from build123d import *

# Parameters (mm, degrees)
F0_W     = 76.2
F0_H     = 25.4
F1_DEPTH = 25.4
F2_W     = 38.1
F2_H     = 25.4
F3_DEPTH = 12.7
F4_R     = 3.175
F5_DEPTH = 12.7


with BuildPart() as f1:
    # F0 (on Front) → F1 (new body)
    with BuildSketch(Plane.XZ):
        with Locations((38.1, 12.7)):
            Rectangle(F0_W, F0_H)
    extrude(amount=F1_DEPTH)

    # F2 (on face) → F3 (cut)
    with BuildSketch(Plane.XY.offset(25.4)):
        with Locations((50.8, -12.7)):
            Rectangle(F2_W, F2_H)
    extrude(amount=-F3_DEPTH, mode=Mode.SUBTRACT)

    # F4 (on face) → F5 (cut)
    with BuildSketch(Plane.XY.offset(12.7)):
        with Locations((43.815, -13.335)):
            Circle(F4_R)
    extrude(amount=-F5_DEPTH, mode=Mode.SUBTRACT)

    # F6: F1 across plane


with BuildPart() as f1_1:
    add(f1.part)
    add(f1.part.mirror(Plane.XY))


solid = f1_1.part
Verification items for the finished model (mm, model axes). A direction names the side the tool comes from. Give positions to 0.01 mm unless a question says otherwise; leave off trailing zeros. Write each loop counter-clockwise with the first axis right and the second up, starting at its lowest first coordinate (ties: lowest second). Pieces come first, ordered by that corner, then holes.
(1) Mould release check, pull along X, two halves, no side actions. Record for faces 4 (the face through (76.2, -13, 0)), 5 (the face through (38, -25.4, 0)), 6 (the face through (51, -13, 12.7)): +X half, -X half, draft (parallel to the pull), parting line (faces both ways), or undercut.
(2) Cross-section at D-D (z = 5.5). Enter the section's corners in (x, y) (3 decimals).
(3) Material ranges on line 1 (Y direction, x = 43.5, z = 11); line 2 (X direction, y = -7, z = 17.5); line 3 (X direction, y = -13.5, z = -7), recorded low to high.
(4) Cross-section at C-C (y = -11). Enter the section's corners in (x, z), plus the area to 3 significant figures.
(5) Gauge pin test, flat ends, axial feed: pin 1 (6 mm diameter, centred on x = 65, y = -20.5, fed in from -Z); pin 2 (12.5 mm diameter, centred on x = 54.5, y = -15, fed in from +Z). Record the tip position at first contact, or that the pin passes through.
(6) Access from +Z, -Z, +X, -X, +Y, -Y to the whole of each face (thin tool, end or side, straight path). Record for faces 1 (the face through (31.75, -13, 19)), 2 (the face through (73, -13, 25.4)), 3 (the face through (51, -13, -12.7)).
(7) Cross-section at A-A (z = -17.5). Enter the section's corners in (x, y), plus the area to 3 significant figures.
(8) Cross-section at B-B (y = -17.5). Enter the section's corners in (x, z).
Worked out:
1. face 4: +X half
1. face 5: draft
1. face 6: undercut
2. outline: (0, -25.4) - (76.2, -25.4) - (76.2, 0) - (0, 0) - close; hole circle Ø6.35 at (43.815, -13.335)
3. line 1: y = -25.4 to -16.49, -10.18 to 0
3. line 2: x = 0 to 31.75, 69.85 to 76.2
3. line 3: x = 0 to 40.64, 46.99 to 76.2
4. outline: (0, -25.4) - (31.75, -25.4) - (31.75, -12.7) - (41.66, -12.7) - (41.66, 12.7) - (31.75, 12.7) - (31.75, 25.4) - (0, 25.4) - close; (45.97, -12.7) - (69.85, -12.7) - (69.85, -25.4) - (76.2, -25.4) - (76.2, 25.4) - (69.85, 25.4) - (69.85, 12.7) - (45.97, 12.7) - close
4. area: 2,790 mm2
5. pin 1: stops at z = -12.7
5. pin 2: stops at z = 12.7
6. face 1: +Z, +Y, -Y
6. face 2: +Z, +X, -X, +Y, -Y
6. face 3: -Z, +Y, -Y
7. outline: (0, -25.4) - (31.75, -25.4) - (31.75, 0) - (0, 0) - close; (69.85, -25.4) - (76.2, -25.4) - (76.2, 0) - (69.85, 0) - close
7. area: 968 mm2
8. outline: (0, -25.4) - (31.75, -25.4) - (31.75, -12.7) - (69.85, -12.7) - (69.85, -25.4) - (76.2, -25.4) - (76.2, 25.4) - (69.85, 25.4) - (69.85, 12.7) - (31.75, 12.7) - (31.75, 25.4) - (0, 25.4) - close
